from build123d import *

# Parameters (mm, degrees)
F0_W           = 1570
F0_H           = 700
F1_DEPTH       = 40
F3_DEPTH       = 100
F4_R           = 75
F5_W           = 30
F5_H           = 30
F6_DEPTH       = 980
F7_W           = 30
F7_H           = 30
F8_DEPTH       = 735
F8_DEPTH_BACK  = 735
F9_W           = 30
F9_H           = 30
F10_DEPTH      = 275
F10_DEPTH_BACK = 245
F11_W          = 30
F11_H          = 30
F12_DEPTH      = 880
F13_W          = 30
F13_H          = 30
F14_DEPTH      = 365
F14_DEPTH_BACK = 350
F15_W          = 30
F15_H          = 30
F16_DEPTH      = 275
F16_DEPTH_BACK = 245
F18_DEPTH      = 2
F20_DEPTH      = 2
F22_DEPTH      = 580
F24_DEPTH      = 580


with BuildPart() as f1:
    # F0 (on Top) → F1 (new body)
    with BuildSketch(Plane.XY):
        Rectangle(F0_W, F0_H)
    extrude(amount=F1_DEPTH)

    # F2 (on face) → F3 (join)
    with BuildSketch(Plane.XY.offset(40)):
        Polygon((-785, 350), (-785, -350), (-783, -350), (-783, 348), (783, 348), (783, -350), (785, -350), (785, 350), align=None)
    extrude(amount=F3_DEPTH)

    # F4
    f4_edges = [f1.edges().sort_by_distance(p)[0] for p in [
        (-784, -350, 140),
        (784, -350, 140),
    ]]
    fillet(f4_edges, radius=F4_R)

    # F5 (on face) → F6 (join)
    with BuildSketch(Plane(origin=(0, 0, 0), x_dir=(1, 0, 0), z_dir=(0, 0, -1))):
        with Locations((-750, 290)):
            Rectangle(F5_W, F5_H)
        with Locations((750, 290)):
            Rectangle(F5_W, F5_H)
        with Locations((750, -260)):
            Rectangle(F5_W, F5_H)
        with Locations((-750, -260)):
            Rectangle(F5_W, F5_H)
    extrude(amount=F6_DEPTH)

    # F7 (on Right) → F8 (join, two sides)
    with BuildSketch(Plane.YZ) as f8_sk:
        with Locations((-290, -895)):
            Rectangle(F7_W, F7_H)
        with Locations((260, -895)):
            Rectangle(F7_W, F7_H)
    extrude(amount=F8_DEPTH)
    extrude(f8_sk.sketch, amount=-F8_DEPTH_BACK)

    # F9 (on Front) → F10 (join, two sides)
    with BuildSketch(Plane.XZ) as f10_sk:
        with Locations((-750, -895)):
            Rectangle(F9_W, F9_H)
        with Locations((750, -895)):
            Rectangle(F9_W, F9_H)
    extrude(amount=F10_DEPTH)
    extrude(f10_sk.sketch, amount=-F10_DEPTH_BACK)

    # F11 (on face) → F12 (join, through all)
    with BuildSketch(Plane(origin=(0, 0, 0), x_dir=(1, 0, 0), z_dir=(0, 0, -1))):
        with Locations((-365, 290)):
            Rectangle(F11_W, F11_H)
        with Locations((380, 290)):
            Rectangle(F11_W, F11_H)
        with Locations((380, -260)):
            Rectangle(F11_W, F11_H)
        with Locations((-365, -260)):
            Rectangle(F11_W, F11_H)
    extrude(amount=F12_DEPTH)

    # F13 (on Right) → F14 (join, two sides)
    with BuildSketch(Plane.YZ) as f14_sk:
        with Locations((-290, -440)):
            Rectangle(F13_W, F13_H)
        with Locations((260, -440)):
            Rectangle(F13_W, F13_H)
    extrude(amount=F14_DEPTH)
    extrude(f14_sk.sketch, amount=-F14_DEPTH_BACK)

    # F15 (on Front) → F16 (join, two sides)
    with BuildSketch(Plane.XZ) as f16_sk:
        with Locations((-365, -440)):
            Rectangle(F15_W, F15_H)
        with Locations((380, -440)):
            Rectangle(F15_W, F15_H)
        with Locations((380, -895)):
            Rectangle(F15_W, F15_H)
        with Locations((-365, -895)):
            Rectangle(F15_W, F15_H)
    extrude(amount=F16_DEPTH)
    extrude(f16_sk.sketch, amount=-F16_DEPTH_BACK)

    # F17 (on face) → F18 (join)
    with BuildSketch(Plane.XY.offset(-425)):
        Polygon((365, 245), (365, 275), (-350, 275), (-350, 245), (-380, 245), (-380, -275), (-350, -275), (-350, -305), (365, -305), (365, -275), (395, -275), (395, 245), align=None)
    extrude(amount=F18_DEPTH)

    # F19 (on face) → F20 (join)
    with BuildSketch(Plane.XY.offset(-880)):
        Polygon((365, 245), (365, 275), (-350, 275), (-350, 245), (-380, 245), (-380, -275), (-350, -275), (-350, -305), (365, -305), (365, -275), (395, -275), (395, 245), align=None)
    extrude(amount=F20_DEPTH)

    # F21 (on face) → F22 (join, through all)
    with BuildSketch(Plane.XZ.offset(305)):
        Polygon((-733, -775), (-735, -775), (-735, -805), (-685, -805), (-685, -803), (-733, -803), align=None)
        Polygon((-735, -573), (-735, -603), (-685, -603), (-685, -601), (-733, -601), (-733, -573), align=None)
        Polygon((-735, -371), (-735, -401), (-685, -401), (-685, -399), (-733, -399), (-733, -371), align=None)
        Polygon((-735, -169), (-735, -199), (-685, -199), (-685, -197), (-733, -197), (-733, -169), align=None)
        Polygon((-430, -803), (-430, -805), (-380, -805), (-380, -775), (-382, -775), (-382, -803), align=None)
        Polygon((-430, -601), (-430, -603), (-380, -603), (-380, -573), (-382, -573), (-382, -601), align=None)
        Polygon((-430, -399), (-430, -401), (-380, -401), (-380, -371), (-382, -371), (-382, -399), align=None)
        Polygon((-380, -169), (-382, -169), (-382, -197), (-430, -197), (-430, -199), (-380, -199), align=None)
    extrude(amount=-F22_DEPTH)

    # F23 (on face) → F24 (join, through all)
    with BuildSketch(Plane.XZ.offset(305)):
        Polygon((397, -700), (395, -700), (395, -730), (425, -730), (425, -728), (397, -728), align=None)
        Polygon((397, -548), (395, -548), (395, -578), (425, -578), (425, -576), (397, -576), align=None)
        Polygon((397, -396), (395, -396), (395, -426), (425, -426), (425, -424), (397, -424), align=None)
        Polygon((397, -244), (395, -244), (395, -274), (425, -274), (425, -272), (397, -272), align=None)
        Polygon((397, -92), (395, -92), (395, -122), (425, -122), (425, -120), (397, -120), align=None)
        Polygon((735, -244), (733, -244), (733, -272), (705, -272), (705, -274), (735, -274), align=None)
        Polygon((735, -92), (733, -92), (733, -120), (705, -120), (705, -122), (735, -122), align=None)
        Polygon((705, -424), (705, -426), (735, -426), (735, -396), (733, -396), (733, -424), align=None)
        Polygon((705, -730), (735, -730), (735, -700), (733, -700), (733, -728), (705, -728), align=None)
        Polygon((735, -578), (735, -548), (733, -548), (733, -576), (705, -576), (705, -578), align=None)
    extrude(amount=-F24_DEPTH)


solid = f1.part
Design review of the part built by this model. Coordinates are the model's own, in mm. A direction names the side the tool comes from. Coordinates: 2 decimals unless noted, no trailing zeros. Order: outer loops, then holes, each group sorted by start corner. A loop starts at its lowest first (then second) coordinate and runs counter-clockwise, first axis right, second up.
Item 1: Take a section at A-A, the plane z = -226. Count the separate pieces of the cut face and the enclosed holes in it, then the cut area to 3 significant figures.
Item 2: Take a section at D-D, the plane x = 301. Write out the cut boundary in (y, z), then the cut area to 3 significant figures.
Item 3: For line 1 (X direction, y = 250, z = -453); line 2 (Z direction, x = 389.5, y = 71); line 3 (Z direction, x = -243.5, y = 240), list the stretches that pass through material, from the lowest coordinate up.
Item 4: The part is to be moulded in two halves that separate along Y. For faces 4 (the flat face through (-60, -305, -451)), 5 (the flat face through (-406, -19, -803)), 6 (the flat face through (395, -14, -880)), 7 (the flat face through (2, -11, -425)), say which applies: pulls with the +Y half, pulls with the -Y half, needs draft (parallel to the pull), parting line crosses it, or undercut.
Item 5: For faces 1 (the flat face through (-406, -19, -399)), 2 (the flat face through (-60, 275, -451)), 3 (the flat face through (-11, 348, 89)), list the 3-axis set-ups (+Z, -Z, +X, -X, +Y, -Y) from which the entire face can be reached by the end or side of a thin tool; tool diameter is ignored.
Item 6: For pin 1 Ø15 at (y, z) = (-293.5, -782) entering from -X; pin 2 Ø3 at (x, y) = (51, -128) entering from -Z; pin 3 Ø15 at (y, z) = (70, -787.5) entering from +X, all flat-tipped, find the tip position at first contact; note any pin that passes through.
Item 7: Take a section at B-B, the plane x = -500.5. Write out the cut boundary in (y, z).
The answers:
1. separate pieces: 8
1. enclosed holes: 0
1. area: 7,200 mm2
2. outline: (-350, 0) - (350, 0) - (350, 140) - (348, 140) - (348, 40) - (-350, 40) - close; (-305, -910) - (-275, -910) - (-275, -880) - (245, -880) - (245, -910) - (275, -910) - (275, -878) - (-305, -878) - close; (-305, -455) - (-275, -455) - (-275, -425) - (245, -425) - (245, -455) - (275, -455) - (275, -423) - (-305, -423) - close
2. area: 34,100 mm2
3. line 1: x = -765 to -735, -380 to 395, 735 to 765
3. line 2: z = -910 to -878, -455 to -423, 0 to 40
3. line 3: z = -880 to -878, -425 to -423, 0 to 40
4. face 4: pulls with the -Y half
4. face 5: needs draft
4. face 6: undercut
4. face 7: undercut
5. face 1: +Y, -Y
5. face 2: -Z, +X, -X, +Y
5. face 3: +Z, -Y
6. pin 1: stops at x = -765
6. pin 2: stops at z = -880
6. pin 3: stops at x = -380
7. outline: (-350, 0) - (350, 0) - (350, 140) - (348, 140) - (348, 40) - (-350, 40) - close; (-305, -910) - (-275, -910) - (-275, -880) - (-305, -880) - close; (245, -910) - (275, -910) - (275, -880) - (245, -880) - close
